The listing builds one solid part. Answer for the finished solid, in the listing's coordinates (mm). A direction names the side the tool comes from. Give positions to 0.01 mm unless a question says otherwise; leave off trailing zeros. Order: outer loops, then holes, each group sorted by start corner. A loop starts at its lowest first (then second) coordinate and runs counter-clockwise, first axis right, second up. Notation, with made-up numbers: (-36.75, 82) - (-0.75, 82) arc R23 cw to (-0.75, 104) - close; hole circle Ø4 at (-17, 89). An arc over 180 degrees is marked (long way). Answer in a Markdown table with one row per item.
from build123d import *

# Parameters (mm, degrees)
F0_W     = 914.4
F0_H     = 609.6
F1_DEPTH = 38.1
F2_W     = 914.4
F2_H     = 609.6
F3_ANGLE = 90
F4_DEPTH = 38.1


with BuildPart() as f1:
    # F0 (on Top) → F1 (new body)
    with BuildSketch(Plane.XY):
        Rectangle(F0_W, F0_H)
    extrude(amount=F1_DEPTH)

    # F2 (on face) → F3 (revolve)
    with BuildSketch(Plane.XY.offset(38.1)):
        Rectangle(F2_W, F2_H)
    revolve(axis=Axis((-103.2055318356, 914.4, 38.1), (-1, 0, 0)), revolution_arc=F3_ANGLE)

    # F4 (add): a face of the model
    f4_faces = [f1.faces().sort_by_distance(p)[0] for p in [
        (0, 914.4, 952.5),
    ]]
    extrude(f4_faces, amount=F4_DEPTH)


solid = f1.part
Item 1: Each of these flat-tipped pins is pushed along its axis until it touches: P1, Ø4, axis at x = -176.5, z = 129, coming from the +Y side; P2, Ø5, axis at x = 247.5, y = 429, coming from the +Z side; P3, Ø5, axis at x = 91, y = 422, coming from the -Z side. Where does it stop, or does it pass through?
Answer block:
| item | result |
|---|---|
| P1 | y = 311.92 |
| P2 | z = 1157.59 |
| P3 | z = 394.03 |
Item 2: Consider line 1 (Y direction, x = 120, z = 150); line 2 (Y direction, x = 251, z = 1016.5); line 3 (Z direction, x = -216.5, y = -114). Determine where each line is inside the solid, lowest interval first.
Answer block:
| item | result |
|---|---|
| line 1 | -299.65 to 315.16 |
| line 2 | 186.95 to 952.5 |
| line 3 | 0 to 692.96 |
Item 3: Find section B-B on y = -156. Write down the section's boundary in (x, z).
Answer block:
| item | result |
|---|---|
| outline | (-457.2, 0) - (457.2, 0) - (457.2, 621.79) - (-457.2, 621.79) - close |
Item 4: Find section C-C on z = 586.5. Write down the section's boundary in (x, y), then the cut area to 3 significant figures.
Answer block:
| item | result |
|---|---|
| outline | (-457.2, -174.5) - (457.2, -174.5) - (457.2, 648.19) - (-457.2, 648.19) - close |
| area | 752,000 mm² |
Item 5: Which of the six approach directions +Z, -Z, +X, -X, +Y, -Y give full straight-line access (tool end or side, diameter ignored) to faces 1 (the face through (-6, 952.5, 948)), 2 (the face through (-6, 933, 647.7))?
Answer block:
| item | result |
|---|---|
| face 1 | +Z, -Z, +X, -X, +Y |
| face 2 | -Z, +X, -X, +Y |
Item 6: Find section A-A on x = 228. Write down the section's boundary in (y, z).
Answer block:
| item | result |
|---|---|
| outline | (-304.8, 0) - (304.8, 0) - (304.8, 38.1) arc R609.6 cw to (914.4, 647.7) - (952.5, 647.7) - (952.5, 1257.3) - (914.4, 1257.3) arc R1219.2 ccw to (-304.8, 38.1) - close |
